from build123d import *

# Parameters (mm, degrees)
SKETCH1_R           = 25
BOSS_EXTRUDE1_DEPTH = 308.600418
SKETCH2_R           = 20.329088143
CUT_EXTRUDE1_DEPTH  = 311.619088257
CHAMFER1_SIZE       = 5.871972
CHAMFER1_SIZE_2     = 3.390185


with BuildPart() as part:
    # Sketch1 → Boss-Extrude1 (new body)
    with BuildSketch(Plane(origin=(0, 0, 0), x_dir=(1, 0, 0), z_dir=(0, 1, 0))):
        with Locations(Location((0, 0, 0), (0, 0, 270))):
            Circle(SKETCH1_R)
    extrude(amount=BOSS_EXTRUDE1_DEPTH)

    # Sketch2 → Cut-Extrude1 (cut, through all)
    with BuildSketch(Plane(origin=(0, 0, 0), x_dir=(1, 0, 0), z_dir=(0, 1, 0))):
        with Locations(Location((0, 0, 0), (0, 0, 270))):
            Circle(SKETCH2_R)
    extrude(amount=CUT_EXTRUDE1_DEPTH, mode=Mode.SUBTRACT)

    # Chamfer1
    # the kernel refuses this chamfer: 5.871972, 3.390185 mm, written as the material it takes off along each edge
    with BuildSketch(Plane(origin=(0, 308.600418, 0), x_dir=(0, 0, 1), z_dir=(-1, 0, 0))) as chamfer1_piece_1:
        Polygon((25, -CHAMFER1_SIZE), (25 - CHAMFER1_SIZE_2, 0), (25, 0), align=None)
    revolve(axis=Axis((0, 308.600418, 0), (0, 1, 0)), mode=Mode.SUBTRACT)
    with BuildSketch(Plane(origin=(0, 0, 0), x_dir=(0, 0, 1), z_dir=(-1, 0, 0))) as chamfer1_piece_2:
        Polygon((25, CHAMFER1_SIZE_2), (25 - CHAMFER1_SIZE, 0), (25, 0), align=None)
    revolve(axis=Axis((0, 0, 0), (0, 1, 0)), mode=Mode.SUBTRACT)


solid = part.part
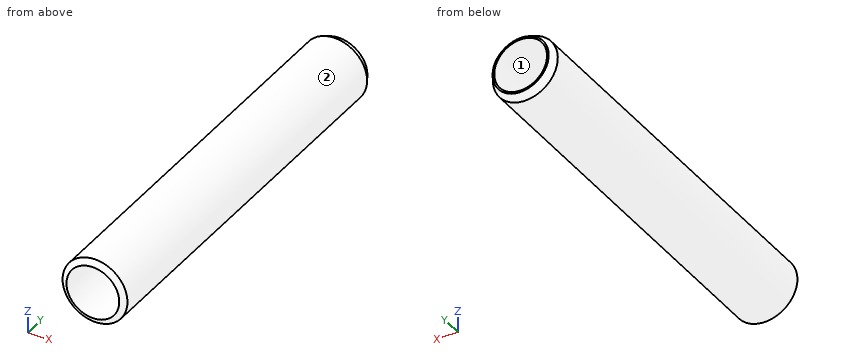
CAD build for the part. Positions are in the model's coordinates, mm. Face numbers are marked on the shaded views. Coordinates: 2 decimals unless noted, no trailing zeros. Write each loop counter-clockwise with the first axis right and the second up, starting at its lowest first coordinate (ties: lowest second). Pieces come first, ordered by that corner, then holes. Notation, with made-up numbers: M -28,82.5 L 26,82.5 A35 ccw 26,119.5 Z; hole C -30.75,73.25 d1. An arc over 180 degrees is marked long. Answer as a JSON object with one key per item and string values. Group by question number.
1) Saw through at B-B (z = 0). Write the cut outline in (x, y), plus the area to 3 significant figures.
2) Pin check, flat tips, straight feed: pin 1 Ø12 at (x, y) = (-18, 191) entering from +Z; pin 2 Ø12 at (x, z) = (-17, -1) entering from -Y; pin 3 Ø6 at (y, z) = (52.5, -17) entering from -X; pin 4 Ø10 at (y, z) = (107, -12) entering from +X. Stop position of each tip, or through.
3) Saw through at A-A (x = 0). Write the cut outline in (y, z).
4) Wall check: line 1 (X direction, y = 55, z = 1.5); line 2 (Z direction, x = -0.5, y = 181) (3 decimals); line 3 (X direction, y = 81.5, z = 3.5). Give the ranges that are in metal, low to high. Write a range as from..to.
5) Saw through at C-C (y = 240). Write the cut outline in (x, z).
6) Mould opens along X. For the marked faces 1 and 2 say: +X half, -X half, draft (parallel to the pull), parting line (faces both ways), or undercut.
Values follow:
{
 "1": {"outline": "M -25,3.39 L -20.33,0.69 L -20.33,308.6 L -21.61,308.6 L -25,302.73 Z; M 20.33,0.69 L 25,3.39 L 25,302.73 L 21.61,308.6 L 20.33,308.6 Z", "area": "2,840 mm2"},
 "2": {"pin 1": "stops at z = 21.93", "pin 2": "stops at y = 0.69", "pin 3": "stops at x = -20.71", "pin 4": "stops at x = 24"},
 "3": {"outline": "M 0.69,-20.33 L 3.39,-25 L 302.73,-25 L 308.6,-21.61 L 308.6,-20.33 Z; M 0.69,20.33 L 308.6,20.33 L 308.6,21.61 L 302.73,25 L 3.39,25 Z"},
 "4": {"line 1": "x = -24.95..-20.27, 20.27..24.95", "line 2": "z = -24.995..-20.323, 20.323..24.995", "line 3": "x = -24.75..-20.03, 20.03..24.75"},
 "5": {"outline": "C 0,0 d50; hole C 0,0 d40.66"},
 "6": {"face 1": "undercut", "face 2": "parting line"}
}
